Can you work these out from the model? Positions are in its coordinate system, mm. Face numbers are marked on the shaded views. Round coordinates to 2 decimals unless told otherwise and drop trailing zeros.
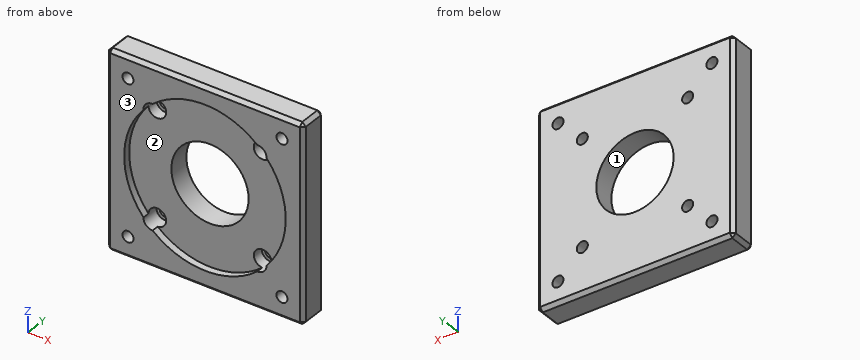
```python
from build123d import *

# Parameters (mm, degrees)
F0_W           = 88.9
F0_H           = 88.9
F0_R           = 2.5
F0_R_2         = 17.4625
F1_DEPTH       = 12.7
F2_R           = 36.5125
F3_DEPTH       = 3.175
F5_D           = 5
F5_START       = 3.175
F5_CBORE_D     = 8
F5_CBORE_DEPTH = 5
F6_SIZE        = 1.5875


with BuildPart() as f1:
    # F0 (on Front) → F1 (new body)
    with BuildSketch(Plane.XZ):
        Rectangle(F0_W, F0_H)
        with Locations((-34.8, -34.8)):
            Circle(F0_R, mode=Mode.SUBTRACT)
        with Locations((34.8, -34.8)):
            Circle(F0_R, mode=Mode.SUBTRACT)
        with Locations((-34.8, 34.8)):
            Circle(F0_R, mode=Mode.SUBTRACT)
        Circle(F0_R_2, mode=Mode.SUBTRACT)
        with Locations((34.8, 34.8)):
            Circle(F0_R, mode=Mode.SUBTRACT)
    extrude(amount=F1_DEPTH)

    # F2 (on face) → F3 (cut)
    with BuildSketch(Plane.XZ.offset(12.7)):
        Circle(F2_R)
    extrude(amount=-F3_DEPTH, mode=Mode.SUBTRACT)

    # F5 (through all)
    # its depths count from where the whole tool has entered the part; down to there all is cleared
    with Locations(Plane.XZ.offset(12.7).offset(-F5_START)):
        with Locations((-23.8125, 23.8125), (23.8125, 23.8125), (23.8125, -23.8125), (-23.8125, -23.8125)):
            CounterBoreHole(F5_D / 2, F5_CBORE_D / 2, F5_CBORE_DEPTH)

    # F6
    f6_edges = [f1.edges().sort_by_distance(p)[0] for p in [
        (0, -12.7, 44.45),
        (-44.45, -12.7, 0),
        (44.45, -12.7, 0),
        (0, -12.7, -44.45),
        (44.45, 0, 0),
        (0, 0, -44.45),
        (-44.45, 0, 0),
        (0, 0, 44.45),
        (-44.45, -6.35, 44.45),
        (-44.45, -6.35, -44.45),
        (44.45, -6.35, 44.45),
        (44.45, -6.35, -44.45),
    ]]
    chamfer(f6_edges, length=F6_SIZE)


solid = f1.part
```
(1) Suppose I cut it at C-C (z = 34.8). Give the number of separate pieces and of enclosed holes in the cut face, then the cut area to 3 significant figures.
(2) For pin 1 (6.5 mm diameter, centred on x = -23.81, z = 23.81, fed in from +Y); pin 2 (21 mm diameter, centred on x = 0, z = 0, fed in from -Y); pin 3 (6.5 mm diameter, centred on x = -24, z = -24, fed in from -Y) (3 decimals); pin 4 (5 mm diameter, centred on x = -8, z = 32, fed in from -Y) (3 decimals), each with a flat end and sliding along its axis, tell me the tip position at first contact or that it passes through.
(3) If I drill on line 1 (Z direction, x = 35, y = -4.75); line 2 (Z direction, x = 23.5, y = -6.75); line 3 (Z direction, x = 0, y = -3.5), over which ranges is the centre line in solid material (lowest first)?
(4) We'd pull the mould along X, two halves only. Please class the marked faces 1, 2 and 3: released by +X, released by -X, zero draft, split by the parting line, or undercut.
Check result:
1. separate pieces: 3
1. enclosed holes: 0
1. area: 927 mm2
2. pin 1: stops at y = 0
2. pin 2: passes through
2. pin 3: stops at y = -4.525
2. pin 4: stops at y = -9.525
3. line 1: z = -44.45 to -37.29, -32.31 to 32.31, 37.29 to 44.45
3. line 2: z = -44.45 to -27.8, -19.82 to 19.82, 27.8 to 44.45
3. line 3: z = -44.45 to -17.46, 17.46 to 44.45
4. face 1: undercut
4. face 2: undercut
4. face 3: zero draft
